For this review, take the finished solid that the model builds, in its own axes (mm). A direction names the side the tool comes from. Coordinates: 2 decimals unless noted, no trailing zeros. Write each loop counter-clockwise with the first axis right and the second up, starting at its lowest first coordinate (ties: lowest second). Pieces come first, ordered by that corner, then holes. Notation, with made-up numbers: (23, -21) - (36, -21) arc R18 cw to (36, -3) - close; hole circle Ø7 at (88.25, -25.75). An arc over 180 degrees is marked (long way). Use one line per item in the form item = value. Start each with the question number.
1) We need section A-A (y = 3.25). Give the boundary of the cut face in (x, z).
2) Insertion check: P1, Ø2.5, axis at x = 39, z = -46, coming from the +Y side; P2, Ø1.8, axis at x = 12.5, y = 1, coming from the -Z side; P3, Ø0.8, axis at y = 0.5, z = 21, coming from the -X side; P4, Ø2.5, axis at x = 40, y = 6.5, coming from the +Z side. Each pin has a flat end and moves straight along its axis. Give the tip position at first contact, or say it passes through.
3) We need section B-B (x = 40). Give the boundary of the cut face in (y, z).
4) Mouldability with a two-part tool opening along Z and no side actions: class faces 1 (the cylindrical face through (26.89, 0.79, -22.51)), 2 (the flat face through (39, 7, -51)), 3 (the flat face through (39, 1.6, -49)) as pulls with the +Z half, pulls with the -Z half, needs draft (parallel to the pull), parting line crosses it, or undercut.
5) We need section C-C (z = -21.5). Give the boundary of the cut face in (x, y).
6) We need section D-D (z = 41.5). Give the boundary of the cut face in (x, y), plus the area to 3 significant figures.
7) For L1, parallel to X at y = 0.45, z = -21.5; L2, parallel to X at y = 1.25, z = 41.5; L3, parallel to Z at x = 28, y = 1.2, list the stretches that pass through material, from the lowest coordinate up. Write a range as from..to.
8) Tool access review of faces 4 (the flat face through (35, 7, -41)), 5 (the flat face through (-85, 8, -40)), 6 (the flat face through (-28, 1.6, -49)): name each direction out of +Z, -Z, +X, -X, +Y, -Y from which nothing blocks a thin tool from reaching the whole face with its end or side.
```python
from build123d import *

# Parameters (mm, degrees)
BOSS_EXTRUDE1_DEPTH      = 1.6
SKETCH2_W                = 115
SKETCH2_H                = 21
BOSS_EXTRUDE2_DEPTH      = 13.6
CUT_EXTRUDE1_OUTLINE_R   = 2.5
CUT_EXTRUDE1_OUTLINE_R_2 = 1.5
CUT_EXTRUDE1_DEPTH       = 1.6
SKETCH5_W                = 9
SKETCH5_H                = 19
BOSS_EXTRUDE3_DEPTH      = 11


# Read off the part's stored shape, not the designer's step: Cut-Extrude1
with BuildPart() as part:
    # Sketch1 (on Top Plane) → Boss-Extrude1 (new body)
    with BuildSketch(Plane(origin=(0, 0, 0), x_dir=(1, 0, 0), z_dir=(0, 1, 0))):
        Polygon((-48, 46.5), (-88, 46.5), (-88, 10.5), (-79, 1.5), (-59, 1.5), (-48, -9.5), (-48, -46.5), (48, -46.5), (48, 46.5), align=None)
    extrude(amount=BOSS_EXTRUDE1_DEPTH)

    # Sketch2 → Boss-Extrude2 (add)
    with BuildSketch(Plane(origin=(0, 1.6, 0), x_dir=(1, 0, 0), z_dir=(0, 1, 0))):
        with Locations((-27.5, 40.5)):
            Rectangle(SKETCH2_W, SKETCH2_H)
    extrude(amount=BOSS_EXTRUDE2_DEPTH)

    # Cut-Extrude1 outline → Cut-Extrude1 (cut)
    with BuildSketch(Plane(origin=(0, 0, 0), x_dir=(1, 0, 0), z_dir=(0, 1, 0))):
        with Locations((40, -41.5)):
            Circle(CUT_EXTRUDE1_OUTLINE_R)
        with Locations((28, 21.5)):
            Circle(CUT_EXTRUDE1_OUTLINE_R_2)
        with Locations((-81, 21.5)):
            Circle(CUT_EXTRUDE1_OUTLINE_R_2)
    extrude(amount=CUT_EXTRUDE1_DEPTH, mode=Mode.SUBTRACT)

    # Sketch5 → Boss-Extrude3 (add)
    with BuildSketch(Plane(origin=(0, 1.6, 0), x_dir=(1, 0, 0), z_dir=(0, 1, 0))):
        with Locations((39.5, 41.5)):
            Rectangle(SKETCH5_W, SKETCH5_H)
    extrude(amount=BOSS_EXTRUDE3_DEPTH)


solid = part.part
```
Determined:
q1.outline = (-85, -51) - (30, -51) - (30, -30) - (-85, -30) - close; (35, -51) - (44, -51) - (44, -32) - (35, -32) - close
q2.P1 = 12.6
q2.P2 = -51
q2.P3 = -48
q2.P4 = -32
q3.outline = (0, -46.5) - (1.6, -46.5) - (1.6, -51) - (12.6, -51) - (12.6, -32) - (1.6, -32) - (1.6, 39) - (0, 39) - close; (0, 44) - (1.6, 44) - (1.6, 46.5) - (0, 46.5) - close
q4.face_1 = undercut
q4.face_2 = pulls with the -Z half
q4.face_3 = needs draft
q5.outline = (-88, 0) - (-82.5, 0) - (-82.5, 1.6) - (-88, 1.6) - close; (-79.5, 0) - (26.5, 0) - (26.5, 1.6) - (-79.5, 1.6) - close; (29.5, 0) - (48, 0) - (48, 1.6) - (29.5, 1.6) - close
q6.outline = (-48, 0) - (37.5, 0) - (37.5, 1.6) - (-48, 1.6) - close; (42.5, 0) - (48, 0) - (48, 1.6) - (42.5, 1.6) - close
q6.area = 146 mm²
q7.L1 = -88..-82.5, -79.5..26.5, 29.5..48
q7.L2 = -48..37.5, 42.5..48
q7.L3 = -46.5..-23, -20..46.5
q8.face_4 = +Z, -Z, +Y
q8.face_5 = +Z, -Z, -X, +Y
q8.face_6 = -Z, +X, -X, -Y
